Part model, mm, in its own coordinate system. Round coordinates to 2 decimals unless told otherwise and drop trailing zeros. Loops run counter-clockwise (first coordinate to the right, second up) from the corner with the lowest first, then second, coordinate; pieces in that order, holes last.
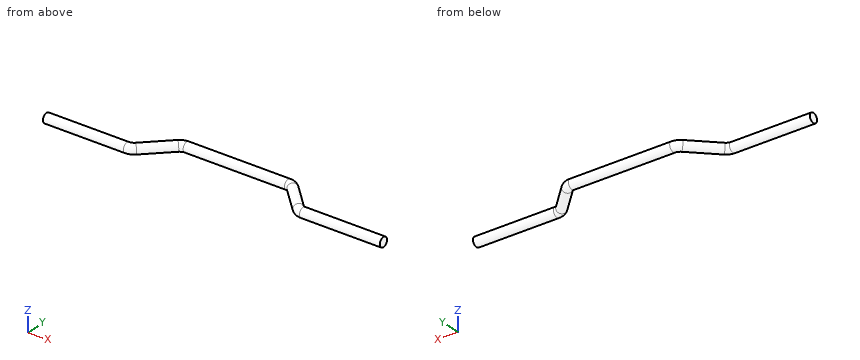
from build123d import *

# Parameters (mm, degrees)
SKETCH2_R = 4


with BuildPart() as part:
    # Base-Sweep: sweep along a path in Sketch1
    with BuildLine(Plane.XY) as base_sweep_path:
        Line((-142.5, -25), (-74.5, -25))
        ThreePointArc((-74.5, -25), (-71.438532541, -24.39103626), (-68.843145751, -22.656854249))
        Line((-68.843145751, -22.656854249), (-48.529437252, -2.343145751))
        ThreePointArc((-48.529437252, -2.343145751), (-45.934050461, -0.60896374), (-42.872583002, 0))
        Line((-42.872583002, 0), (42.872583002, 0))
        ThreePointArc((42.872583002, 0), (45.934050461, -0.60896374), (48.529437252, -2.343145751))
        Line((48.529437252, -2.343145751), (68.843145751, -22.656854249))
        ThreePointArc((68.843145751, -22.656854249), (71.438532541, -24.39103626), (74.5, -25))
        Line((74.5, -25), (142.5, -25))
    # Sketch2 → Base-Sweep (sweep)
    with BuildSketch(Plane(origin=(-142.5, -25, 0), x_dir=(0, 0, 1), z_dir=(-1, 0, 0))):
        Circle(SKETCH2_R)
    sweep(path=base_sweep_path.line)


solid = part.part
1) Slice it at B-B, the plane x = 93. Give the cut face in (y, z).
Values:
outline: circle Ø8 at (-25, 0)
2) Drop flat-ended pins along their axis: pin 1 Ø2 at (y, z) = (-10.5, -2.5) entering from -X; pin 2 Ø1 at (y, z) = (-7, 2.5) entering from -X; pin 3 Ø3 at (x, z) = (93, -2.5) entering from -Y. Give the stop position or say it passes through.
Values:
pin 1: stops at x = -62.46
pin 2: stops at x = -58.31
pin 3: stops at y = -28.87
3) Slice it at A-A, the plane z = 0. Give the cut face in (x, y), then the cut area to 3 significant figures.
Values:
outline: (-142.5, -29) - (-74.5, -29) arc R12 ccw to (-66.01, -25.49) - (-45.7, -5.17) arc R4 cw to (-42.87, -4) - (42.87, -4) arc R4 cw to (45.7, -5.17) - (66.01, -25.49) arc R12 ccw to (74.5, -29) - (142.5, -29) - (142.5, -21) - (74.5, -21) arc R4 cw to (71.67, -19.83) - (51.36, 0.49) arc R12 ccw to (42.87, 4) - (-42.87, 4) arc R12 ccw to (-51.36, 0.49) - (-71.67, -19.83) arc R4 cw to (-74.5, -21) - (-142.5, -21) - close
area: 2,430 mm2
4) Wall check: line 1 along X through (y, z) = (-24, -3.25); line 2 along X through (y, z) = (-15.5, 2.5); line 3 along Z through (x, y) = (-58.5, -11.5). Give the ranges that are in metal, low to high.
Values:
line 1: x = -142.5 to -66.89, 66.89 to 142.5
line 2: x = -66.1 to -57.27, 57.27 to 66.1
line 3: z = -3.96 to 3.96
